The drawing under review shows one solid part. Ordinate dimensions are in mm from its lowest x, y, z. Round coordinates to 2 decimals unless told otherwise and drop trailing zeros. Order: outer loops, then holes, each group sorted by start corner. A loop starts at its lowest first (then second) coordinate and runs counter-clockwise, first axis right, second up. Notation, with made-up numbers: M -4,17 L 43,17 A22 cw 43,44 Z; hole C 63.25,-21 d7. An arc over 180 degrees is marked long. Answer as a JSON object with one key per item and string values. Group by question number.
1) To check wall thickness, follow line 1 (Z direction, x = 63, y = 4.25) (1 decimal); line 2 (Z direction, x = 208, y = 6.25) (1 decimal); line 3 (X direction, y = 4.75, z = 25) (1 decimal). State the ranges of each line that lie inside material, in increasing order.
2) Insertion check: pin 1 Ø1.9 at (x, y) = (129, 3) entering from +Z. The pin has a flat end and moves straight along its axis. Give the tip position at first contact, or say it passes through.
3) Consider section C-C, the plane z = 104.5. Write out the cut boundary in (x, y), then the cut area to 3 significant figures.
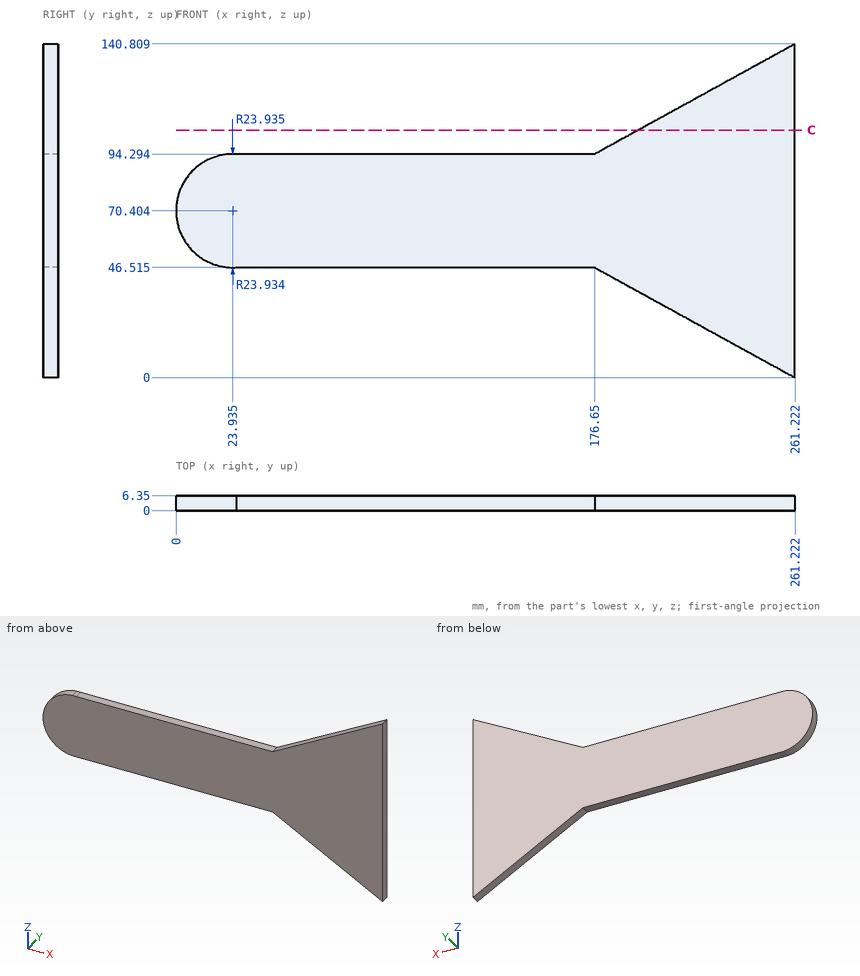
Results list:
{
 "1": {"line 1": "46.5 to 94.3", "line 2": "29.3 to 111.5", "line 3": "215.8 to 261.2"},
 "2": {"pin 1": "z = 94.29"},
 "3": {"outline": "M 195.21,0 L 261.22,0 L 261.22,6.35 L 195.21,6.35 Z", "area": "419 mm^2"}
}
